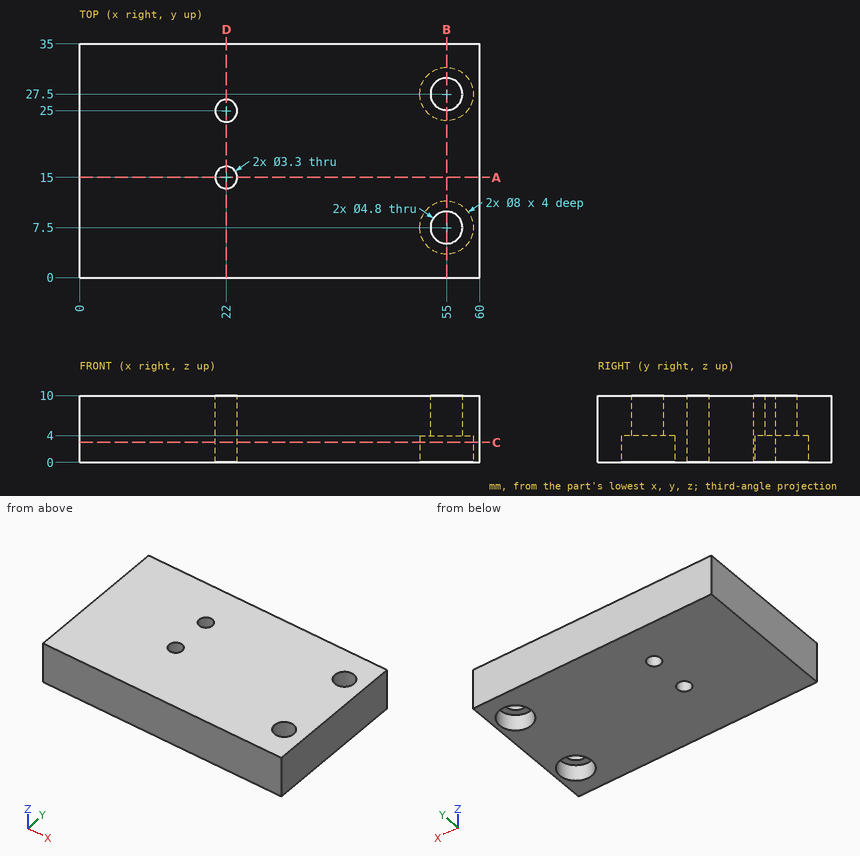
Geometry: see drawing. Coordinates: mm, zero at the bounding-box minimum. Round coordinates to 2 decimals unless told otherwise and drop trailing zeros. Write each loop counter-clockwise with the first axis right and the second up, starting at its lowest first coordinate (ties: lowest second). Pieces come first, ordered by that corner, then holes. Notation, with made-up numbers: M -39.5,50.5 L 13.5,50.5 A8 ccw 13.5,60.5 Z; hole C -21.75,-27 d9. An arc over 180 degrees is marked long. Answer as a JSON object with one key per item and string values. Group by question number.
(1) Section query B-B on x = 55. Output: boundary loops of the cut face in (y, z), then the cut area to 3 significant figures.
(2) Ray query, line 1 (Y direction, x = 55, z = 2.5); line 2 (Y direction, x = 55, z = 7); line 3 (X direction, y = 9, z = 6). Return the intervals inside material, ascending. Write a range as [from, to].
(3) Section query C-C on z = 3. Output: boundary loops of the cut face in (x, y).
(4) Section query D-D on x = 22. Output: boundary loops of the cut face in (y, z).
(5) Section query A-A on y = 15. Output: boundary loops of the cut face in (x, z), then the cut area to 3 significant figures.
(6) First-contact query: pin 1 (7 mm diameter, centred on x = 55, y = 27.5, fed in from -Z). Flat tip, straight axial feed; report the tip coordinate or a pass-through.
Computed values:
{
 "1": {"outline": "M 0,0 L 3.5,0 L 3.5,4 L 5.1,4 L 5.1,10 L 0,10 Z; M 9.9,4 L 11.5,4 L 11.5,0 L 23.5,0 L 23.5,4 L 25.1,4 L 25.1,10 L 9.9,10 Z; M 29.9,4 L 31.5,4 L 31.5,0 L 35,0 L 35,10 L 29.9,10 Z", "area": "228 mm^2"},
 "2": {"line 1": "[0, 3.5], [11.5, 23.5], [31.5, 35]", "line 2": "[0, 5.1], [9.9, 25.1], [29.9, 35]", "line 3": "[0, 53.13], [56.87, 60]"},
 "3": {"outline": "M 0,0 L 60,0 L 60,35 L 0,35 Z; hole C 22,15 d3.3; hole C 22,25 d3.3; hole C 55,7.5 d8; hole C 55,27.5 d8"},
 "4": {"outline": "M 0,0 L 13.35,0 L 13.35,10 L 0,10 Z; M 16.65,0 L 23.35,0 L 23.35,10 L 16.65,10 Z; M 26.65,0 L 35,0 L 35,10 L 26.65,10 Z"},
 "5": {"outline": "M 0,0 L 20.35,0 L 20.35,10 L 0,10 Z; M 23.65,0 L 60,0 L 60,10 L 23.65,10 Z", "area": "567 mm^2"},
 "6": {"pin 1": "z = 4"}
}
